```python
from build123d import *

# Parameters (mm, degrees)
ESBO_O1_R                  = 17.5
ESBO_O1_R_2                = 12.5
RESSALTO_EXTRUS_O1_DEPTH   = 55.6
RESSALTO_EXTRUS_O2_START   = -5
ESBO_O2_R                  = 12.5
RESSALTO_EXTRUS_O2_DEPTH   = 5
RESSALTO_EXTRUS_O3_START   = -34.8
ESBO_O4_R                  = 17.5
ESBO_O4_R_2                = 12.1
RESSALTO_EXTRUS_O3_DEPTH   = 34.8
CORTE_EXTRUS_O4_START      = -5
CORTE_EXTRUS_O4_DEPTH      = 5
ESBO_O13_R                 = 2
CORTE_EXTRUS_O6_DEPTH      = 78
ESBO_O14_W                 = 20
ESBO_O14_H                 = 3
RESSALTO_EXTRUS_O5_DEPTH   = 50.6
CORTE_EXTRUS_O7_DEPTH      = 50.6
CORTE_EXTRUS_O7_DEPTH_BACK = 50.6
ESBO_O15_R                 = 3
ESBO_O19_W                 = 3.249347661
ESBO_O19_H                 = 3
ESBO_O19_W_2               = 1.024720198
CORTE_EXTRUS_O8_DEPTH      = 78
ESBO_O24_W                 = 3
ESBO_O24_H                 = 3
CORTE_EXTRUS_O9_DEPTH      = 78
ESBO_O27_R                 = 4.25
CORTE_EXTRUS_O10_DEPTH     = 10
RESSALTO_EXTRUS_O6_START   = -5
ESBO_O28_R                 = 2
RESSALTO_EXTRUS_O6_DEPTH   = 5
ESBO_O29_R                 = 0.9
CORTE_EXTRUS_O11_DEPTH     = 5


with BuildPart() as part:
    # Esboço1 → Ressalto-extrusão1 (new body)
    with BuildSketch(Plane.XY):
        Circle(ESBO_O1_R)
        Circle(ESBO_O1_R_2, mode=Mode.SUBTRACT)
    extrude(amount=RESSALTO_EXTRUS_O1_DEPTH)

    # Esboço2 → Ressalto-extrusão2 (add)
    with BuildSketch(Plane.XY.offset(55.6).offset(RESSALTO_EXTRUS_O2_START)):
        Circle(ESBO_O2_R)
    extrude(amount=RESSALTO_EXTRUS_O2_DEPTH)

    # Esboço4 → Ressalto-extrusão3 (add)
    with BuildSketch(Plane.XY.offset(55.6).offset(RESSALTO_EXTRUS_O3_START)):
        Circle(ESBO_O4_R)
        Circle(ESBO_O4_R_2, mode=Mode.SUBTRACT)
    extrude(amount=RESSALTO_EXTRUS_O3_DEPTH)

    # Esboço12 → Corte-extrusão4 (cut)
    with BuildSketch(Plane.XY.offset(55.6).offset(CORTE_EXTRUS_O4_START)):
        with BuildLine():
            Line((0, 1.5), (17.435595774, 1.5))
            ThreePointArc((17.435595774, 1.5), (17.5, 0), (17.435595774, -1.5))
            Line((17.435595774, -1.5), (0, -1.5))
            Line((0, -1.5), (-17.435595774, -1.5))
            ThreePointArc((-17.435595774, -1.5), (-17.5, 0), (-17.435595774, 1.5))
            Line((-17.435595774, 1.5), (0, 1.5))
        make_face()
    extrude(amount=CORTE_EXTRUS_O4_DEPTH, mode=Mode.SUBTRACT)

    # Esboço13 → Corte-extrusão6 (cut)
    with BuildSketch(Plane.XY):
        with Locations((0, -7.714268488)):
            Circle(ESBO_O13_R)
    extrude(amount=CORTE_EXTRUS_O6_DEPTH, mode=Mode.SUBTRACT)

    # Esboço14 → Ressalto-extrusão5 (add)
    with BuildSketch(Plane(origin=(0, 0, 50.6), x_dir=(-1, 0, 0), z_dir=(0, 0, -1))):
        with Locations((24.721130295, -4)):
            Rectangle(ESBO_O14_W, ESBO_O14_H)
        with Locations((24.721130295, 4)):
            Rectangle(ESBO_O14_W, ESBO_O14_H)
        with Locations((-24.721130295, 4)):
            Rectangle(ESBO_O14_W, ESBO_O14_H)
        with Locations((-24.721130295, -4)):
            Rectangle(ESBO_O14_W, ESBO_O14_H)
    extrude(amount=RESSALTO_EXTRUS_O5_DEPTH)

    # Esboço15 → Corte-extrusão7 (cut, two sides: drawn at the far end of the back side and taken through both)
    with BuildSketch(Plane(origin=(0, 0, 0), x_dir=(1, 0, 0), z_dir=(0, 1, 0)).offset(-CORTE_EXTRUS_O7_DEPTH_BACK)):
        with Locations((-25.721130295, -25.3)):
            Circle(ESBO_O15_R)
        with Locations((25.721130295, -25.3)):
            Circle(ESBO_O15_R)
        with Locations((-25.721130295, -37.95)):
            Circle(ESBO_O15_R)
        with Locations((-25.721130295, -12.65)):
            Circle(ESBO_O15_R)
        with Locations((25.721130295, -12.65)):
            Circle(ESBO_O15_R)
        with Locations((25.721130295, -37.95)):
            Circle(ESBO_O15_R)
    extrude(amount=CORTE_EXTRUS_O7_DEPTH + CORTE_EXTRUS_O7_DEPTH_BACK, mode=Mode.SUBTRACT)

    # Esboço19 → Corte-extrusão8 (cut)
    with BuildSketch(Plane(origin=(0, 0, 50.6), x_dir=(-1, 0, 0), z_dir=(0, 0, -1))):
        with Locations((19.060269605, 0)):
            Rectangle(ESBO_O19_W, ESBO_O19_H)
        with Locations((-17.947955873, 0)):
            Rectangle(ESBO_O19_W_2, ESBO_O19_H)
    extrude(amount=CORTE_EXTRUS_O8_DEPTH, mode=Mode.SUBTRACT)

    # Esboço24 → Corte-extrusão9 (cut)
    with BuildSketch(Plane(origin=(0, 0, 0), x_dir=(-1, 0, 0), z_dir=(0, 0, -1))):
        with Locations((-15.935595774, 0)):
            Rectangle(ESBO_O24_W, ESBO_O24_H)
        with Locations((15.935595774, 0)):
            Rectangle(ESBO_O24_W, ESBO_O24_H)
    extrude(amount=-CORTE_EXTRUS_O9_DEPTH, mode=Mode.SUBTRACT)

    # Esboço27 → Corte-extrusão10 (cut)
    with BuildSketch(Plane.XY.offset(55.6)):
        Circle(ESBO_O27_R)
    extrude(amount=-CORTE_EXTRUS_O10_DEPTH, mode=Mode.SUBTRACT)

    # Esboço28 → Ressalto-extrusão6 (add)
    with BuildSketch(Plane.XY.offset(55.6).offset(RESSALTO_EXTRUS_O6_START)):
        with Locations((0, -7.714268488)):
            Circle(ESBO_O28_R)
    extrude(amount=RESSALTO_EXTRUS_O6_DEPTH)

    # Esboço29 → Corte-extrusão11 (cut)
    with BuildSketch(Plane.XY.offset(55.6)):
        with Locations((0, 8.5)):
            Circle(ESBO_O29_R)
        with Locations((0, -8.5)):
            Circle(ESBO_O29_R)
    extrude(amount=-CORTE_EXTRUS_O11_DEPTH, mode=Mode.SUBTRACT)


solid = part.part
```
Input: part model. Units: mm. Frame: model coordinates. A direction names the side the tool comes from. Give positions to 0.01 mm unless a question says otherwise; leave off trailing zeros. Order: outer loops, then holes, each group sorted by start corner. A loop starts at its lowest first (then second) coordinate and runs counter-clockwise, first axis right, second up. Notation, with made-up numbers: (20.25, 0.5) - (25.25, 0.5) arc R13 ccw to (25.25, 23.5) - close; hole circle Ø10 at (81, 64). An arc over 180 degrees is marked (long way). One line per item, written item: value.
1. Cut plane A-A, the plane y = 0. Output: boundary loops of the cut face in (x, z), and give its area (3 significant figures).
Determined:
outline: (-14.44, 0) - (-12.5, 0) - (-12.5, 20.8) - (-12.1, 20.8) - (-12.1, 50.6) - (-14.44, 50.6) - close; (12.1, 20.8) - (12.5, 20.8) - (12.5, 0) - (14.44, 0) - (14.44, 50.6) - (12.1, 50.6) - close
area: 220 mm2
2. Draft query along Z for faces 1 (the face through (-26, 4, 50.6)), 2 (the face through (0.07, 4.25, 53.14)), 3 (the face through (-24.11, -4.02, 22.77)). Return one class per face: released by +Z, released by -Z, zero draft, split by the parting line, or undercut.
Determined:
face 1: released by +Z
face 2: zero draft
face 3: undercut
3. Line query: probe 1 along X at (y, z) = (0, 38); probe 2 along X at (y, z) = (-4.5, 25); probe 3 along Y at (x, z) = (-19.5, 42.5). Output: solid intervals per line, ascending.
Determined:
probe 1: -14.44 to -12.1, 12.1 to 14.44
probe 2: -34.72 to -28.71, -22.74 to -11.23, 11.23 to 22.74, 28.71 to 34.72
probe 3: -5.5 to -2.5, 2.5 to 5.5
4. Reachability of faces 4 (the face through (-22, 2.5, 26)), 5 (the face through (23.51, -4.02, 10.62)), 6 (the face through (11.18, -4.63, 35.49)), 7 (the face through (-0.07, -4.25, 53.14)), 8 (the face through (14.436, 0, 25)) from +Z, -Z, +X, -X, +Y, -Y: full face, straight path, thin tool, end or side. Return the list, or none.
Determined:
face 4: +Z, -Z, -X
face 5: +Y, -Y
face 6: -Z
face 7: +Z, -Z
face 8: +Z, -Z, +X
5. Cut plane D-D, the plane x = 11. Output: boundary loops of the cut face in (y, z), and give its area (3 significant figures).
Determined:
outline: (-13.61, 0) - (-5.94, 0) - (-5.94, 20.8) - (-5.04, 20.8) - (-5.04, 50.6) - (-1.5, 50.6) - (-1.5, 55.6) - (-13.61, 55.6) - close; (1.5, 50.6) - (5.04, 50.6) - (5.04, 20.8) - (5.94, 20.8) - (5.94, 0) - (13.61, 0) - (13.61, 55.6) - (1.5, 55.6) - close
area: 951 mm2
6. Pin query (flat end, axial travel): pin 1 Ø6 at (x, z) = (-25, 17) entering from -Y; pin 2 Ø0.7 at (x, y) = (13, 0.5) entering from +Z; pin 3 Ø9.5 at (x, z) = (25.72, 12.65) entering from +Y. Return the tip coordinate at first contact, or that it passes through.
Determined:
pin 1: y = -5.5
pin 2: z = 50.6
pin 3: y = 5.5
7. Cut plane B-B, the plane z = 25.3. Give the number of separate pieces and of enclosed holes in the cut face, and give its area (3 significant figures).
Determined:
separate pieces: 5
enclosed holes: 1
area: 624 mm2
